from build123d import *

# Parameters (mm, degrees)
F0_R     = 254
F1_DEPTH = 215.9
F2_R     = 50.8
F3_DEPTH = 215.901
F4_R     = 189.621559
F5_DEPTH = 48.26


with BuildPart() as f1:
    # F0 (on Front) → F1 (new body)
    with BuildSketch(Plane.XZ):
        Circle(F0_R)
    extrude(amount=F1_DEPTH)

    # F2 (on face) → F3 (cut, through all)
    with BuildSketch(Plane.XZ.offset(215.9)):
        Circle(F2_R)
    extrude(amount=-F3_DEPTH, mode=Mode.SUBTRACT)

    # F4 (on face) → F5 (cut)
    with BuildSketch(Plane.XZ.offset(215.9)):
        Circle(F4_R)
    extrude(amount=-F5_DEPTH, mode=Mode.SUBTRACT)


solid = f1.part
CAD build for the part. Positions are in the model's coordinates, mm. A direction names the side the tool comes from. Coordinates: 2 decimals unless noted, no trailing zeros. Order: outer loops, then holes, each group sorted by start corner. A loop starts at its lowest first (then second) coordinate and runs counter-clockwise, first axis right, second up.
Item 1: Band-saw the part on D-D on z = -86. List the corners of the cut face in (x, y), plus the area to 3 significant figures.
Check sheet entries:
outline: (-239, -215.9) - (-169, -215.9) - (-169, -167.64) - (169, -167.64) - (169, -215.9) - (239, -215.9) - (239, 0) - (-239, 0) - close
area: 86,900 mm2
Item 2: Band-saw the part on C-C on x = 65.5. List the corners of the cut face in (y, z).
Check sheet entries:
outline: (-215.9, -245.41) - (0, -245.41) - (0, 245.41) - (-215.9, 245.41) - (-215.9, 177.95) - (-167.64, 177.95) - (-167.64, -177.95) - (-215.9, -177.95) - close
Item 3: Band-saw the part on A-A on x = 0. List the corners of the cut face in (y, z), plus the area to 3 significant figures.
Check sheet entries:
outline: (-215.9, -254) - (0, -254) - (0, -50.8) - (-167.64, -50.8) - (-167.64, -189.62) - (-215.9, -189.62) - close; (-215.9, 189.62) - (-167.64, 189.62) - (-167.64, 50.8) - (0, 50.8) - (0, 254) - (-215.9, 254) - close
area: 74,300 mm2
Item 4: Drill centre lines: L1, parallel to Z at x = 0, y = -192; L2, parallel to Z at x = 0, y = -62; L3, parallel to Y at x = -176.5, z = 12.5. Where is each one in solid material? Low to high.
Check sheet entries:
L1: z = -254 to -189.62, 189.62 to 254
L2: z = -254 to -50.8, 50.8 to 254
L3: y = -167.64 to 0
Item 5: 3-axis set-ups, long thin cutter, end or side, ignore diameter. For faces 4 (the face through (39, -167.64, -39)), 5 (the face through (-11.012, -84.993, -49.592)): which of +Z, -Z, +X, -X, +Y, -Y reach the whole face in a straight line?
Check sheet entries:
face 4: -Y
face 5: +Y, -Y
Item 6: Band-saw the part on B-B on z = 0. List the corners of the cut face in (x, y).
Check sheet entries:
outline: (-254, -215.9) - (-189.62, -215.9) - (-189.62, -167.64) - (-50.8, -167.64) - (-50.8, 0) - (-254, 0) - close; (50.8, -167.64) - (189.62, -167.64) - (189.62, -215.9) - (254, -215.9) - (254, 0) - (50.8, 0) - close
Item 7: Two-plate mould, pull along Z, no slides. Class faces 1 (the face through (53, 0, 4)), 2 (the face through (-150.48, -192.11, -115.38)), 3 (the face through (-55.06, -106.44, -247.96)): +Z half, -Z half, draft (parallel to the pull), parting line (faces both ways), or undercut.
Check sheet entries:
face 1: draft
face 2: undercut
face 3: parting line
Item 8: Pin check, flat tips, straight feed: pin 1 Ø5 at (y, z) = (-37, 159.5) entering from -X; pin 2 Ø1.5 at (y, z) = (-101, -9) entering from +X; pin 3 Ø1 at (x, y) = (-113.5, -35) entering from -Z. Stop position of each tip, or through.
Check sheet entries:
pin 1: stops at x = -199.67
pin 2: stops at x = 253.87
pin 3: stops at z = -227.48
